Geometry: see drawing. Coordinates: mm, zero at the bounding-box minimum. Coordinates: 2 decimals unless noted, no trailing zeros. Order: outer loops, then holes, each group sorted by start corner. A loop starts at its lowest first (then second) coordinate and runs counter-clockwise, first axis right, second up. Notation, with made-up numbers: (-21, 36.5) - (2, 36.5) arc R9 cw to (2, 53.5) - close; hole circle Ø8 at (65, 4.5). An arc over 180 degrees is marked (long way). Use a Markdown table: item, result. Add a question column.
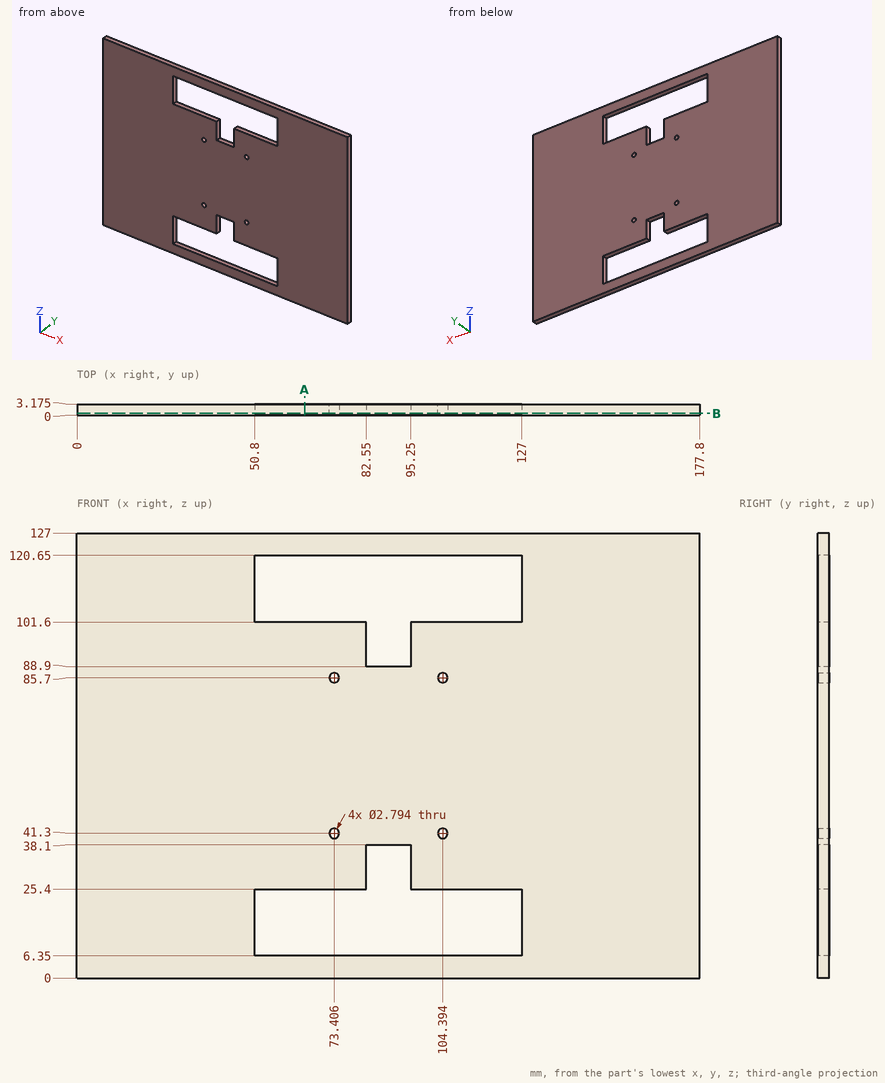
1) Cut plane B-B (y = 0.5). Return the cut outline in (x, z), and give its area (3 significant figures).
2) Material intervals for L1, parallel to Z at x = 88.5, y = 1.45; L2, parallel to Z at x = 61.5, y = 0.7; L3, parallel to X at y = 0.45, z = 86, sorted ascending.
3) Contact query for a flat-ended pin moving along its axis: P1, Ø2, axis at x = 104.39, z = 85.7, coming from the -Y side. Output: stop coordinate, or through.
4) Cut plane A-A (x = 65). State how many separate pieces and enclosed holes the cut face has, and give its area (3 significant figures).
Computed:
| question | item | result |
|---|---|---|
| 1 | outline | (0, 0) - (177.8, 0) - (177.8, 127) - (0, 127) - close; hole (50.8, 6.35) - (127, 6.35) - (127, 25.4) - (95.25, 25.4) - (95.25, 38.1) - (82.55, 38.1) - (82.55, 25.4) - (50.8, 25.4) - close; hole (50.8, 101.6) - (82.55, 101.6) - (82.55, 88.9) - (95.25, 88.9) - (95.25, 101.6) - (127, 101.6) - (127, 120.65) - (50.8, 120.65) - close; hole circle Ø2.79 at (73.41, 41.3); hole circle Ø2.79 at (73.41, 85.7); hole circle Ø2.79 at (104.39, 41.3); hole circle Ø2.79 at (104.39, 85.7) |
| 1 | area | 19,300 mm2 |
| 2 | L1 | z = 0 to 6.35, 38.1 to 88.9, 120.65 to 127 |
| 2 | L2 | z = 0 to 6.35, 25.4 to 101.6, 120.65 to 127 |
| 2 | L3 | x = 0 to 72.04, 74.77 to 103.03, 105.76 to 177.8 |
| 3 | P1 | passes through |
| 4 | separate pieces | 3 |
| 4 | enclosed holes | 0 |
| 4 | area | 282 mm2 |
